Design review of the part built by this model. Coordinates are the model's own, in mm. A direction names the side the tool comes from. Coordinates: 2 decimals unless noted, no trailing zeros. Order: outer loops, then holes, each group sorted by start corner. A loop starts at its lowest first (then second) coordinate and runs counter-clockwise, first axis right, second up. Notation, with made-up numbers: M 55.25,79 L 81.25,79 A11 ccw 81.25,84 Z; hole C 52,68 d1. An arc over 180 degrees is marked long. Answer as a JSON object with one key per item and string values.
from build123d import *

# Parameters (mm, degrees)
SKETCH1_R           = 1.6
BOSS_EXTRUDE2_DEPTH = 5
SKETCH2_W           = 5.53954597
SKETCH2_H           = 8
BOSS_EXTRUDE3_DEPTH = 1.5
SKETCH3_W           = 5.53954597
SKETCH3_H           = 8
BOSS_EXTRUDE4_DEPTH = 1.5


with BuildPart() as part:
    # Sketch1 → Boss-Extrude2 (new body)
    with BuildSketch(Plane.XY):
        with BuildLine():
            Line((0, 4), (-10, 4))
            Line((-10, 4), (-10, -4))
            Line((-10, -4), (0, -4))
            ThreePointArc((0, -4), (4, 0), (0, 4))
        make_face()
        Circle(SKETCH1_R, mode=Mode.SUBTRACT)
    extrude(amount=BOSS_EXTRUDE2_DEPTH)

    # Sketch2 → Boss-Extrude3 (add)
    with BuildSketch(Plane.XY.offset(5)):
        with Locations((-7.230227015, 0)):
            Rectangle(SKETCH2_W, SKETCH2_H)
    extrude(amount=BOSS_EXTRUDE3_DEPTH)

    # Sketch3 → Boss-Extrude4 (add)
    with BuildSketch(Plane(origin=(0, 0, 0), x_dir=(-1, 0, 0), z_dir=(0, 0, -1))):
        with Locations((7.230227015, 0)):
            Rectangle(SKETCH3_W, SKETCH3_H)
    extrude(amount=BOSS_EXTRUDE4_DEPTH)


solid = part.part
1) Add section C-C (y = 1.75). State the section outline as (x, z) points, and give its area (3 significant figures).
Taken from the geometry:
{"outline": "M -10,-1.5 L -4.46,-1.5 L -4.46,0 L 3.6,0 L 3.6,5 L -4.46,5 L -4.46,6.5 L -10,6.5 Z", "area": "84.6 mm2"}
2) Tool access review of faces 4 (the cylindrical face through (4, 0, 2)), 5 (the flat face through (-4.46, 0, -1)), 6 (the flat face through (-4.46, 0, 6)): name each direction out of +Z, -Z, +X, -X, +Y, -Y from which nothing blocks a thin tool from reaching the whole face with its end or side.
Taken from the geometry:
{"face 4": "+Z, -Z, +X", "face 5": "-Z, +X, +Y, -Y", "face 6": "+Z, +X, +Y, -Y"}
3) Add section A-A (y = 0). State the section outline as (x, z) points.
Taken from the geometry:
{"outline": "M -10,-1.5 L -4.46,-1.5 L -4.46,0 L -1.6,0 L -1.6,5 L -4.46,5 L -4.46,6.5 L -10,6.5 Z; M 1.6,0 L 4,0 L 4,5 L 1.6,5 Z"}
4) To check wall thickness, follow L1, parallel to Z at x = 1, y = -3; L2, parallel to Y at x = -1, z = 3; L3, parallel to X at y = -2, z = 5.25. State the ranges of each line that lie inside material, in increasing order.
Taken from the geometry:
{"L1": "z = 0 to 5", "L2": "y = -4 to -1.25, 1.25 to 4", "L3": "x = -10 to -4.46"}
5) Mouldability with a two-part tool opening along X and no side actions: class faces 1 (the flat face through (-6, -4, 3)), 2 (the cylindrical face through (-1.27, -0.97, 2.46)), 3 (the flat face through (-10, 0, 3)) as released by +X, released by -X, zero draft, split by the parting line, or undercut.
Taken from the geometry:
{"face 1": "zero draft", "face 2": "undercut", "face 3": "released by -X"}
6) Insertion check: pin 1 Ø1.2 at (y, z) = (-1, -1) entering from +X; pin 2 Ø4 at (x, y) = (0.5, 0) entering from +Z; pin 3 Ø4 at (x, y) = (-1.5, 0) entering from -Z. Each pin has a flat end and moves straight along its axis. Give the tip position at first contact, or say it passes through.
Taken from the geometry:
{"pin 1": "stops at x = -4.46", "pin 2": "stops at z = 5", "pin 3": "stops at z = 0"}
7) Add section B-B (z = 0.5). State the section outline as (x, y) points.
Taken from the geometry:
{"outline": "M -10,-4 L 0,-4 A4 ccw 0,4 L -10,4 Z; hole C 0,0 d3.2"}
8) Add section D-D (x = -2.25). State the section outline as (y, z) points.
Taken from the geometry:
{"outline": "M -4,0 L 4,0 L 4,5 L -4,5 Z"}
